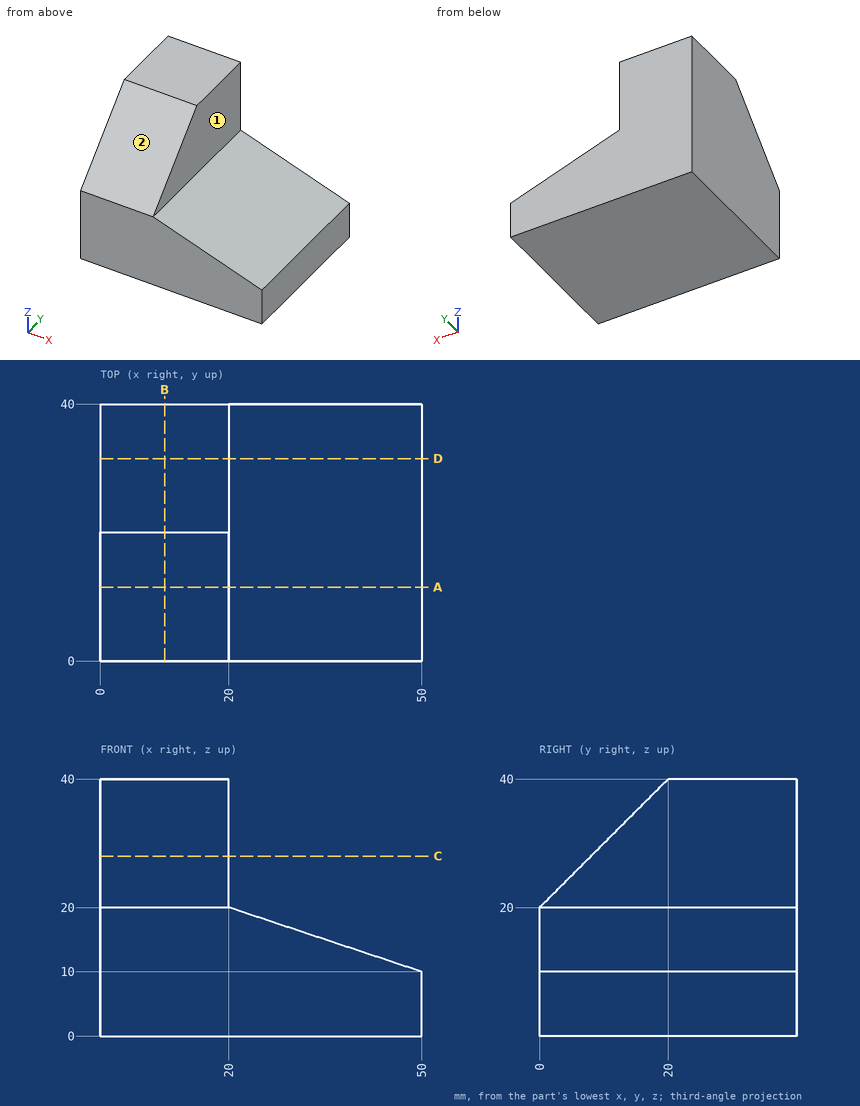
Drawing for the job (mm, zero at the part's lowest x, y, z). A direction names the side the tool comes from. Give positions to 0.01 mm unless a question says otherwise; leave off trailing zeros. Write each loop counter-clockwise with the first axis right and the second up, starting at its lowest first coordinate (ties: lowest second). Pieces come first, ordered by that corner, then holes. Notation, with made-up numbers: (11.25, 40.25) -> (38.25, 40.25) arc R4 cw to (38.25, 46.25) -> close; hole circle Ø1 at (11, 75.25). An arc over 180 degrees is marked (long way). Put each result on its own line as item: value. Start each with the question number.
Item 1: Which spindle directions (+Z, -Z, +X, -X, +Y, -Y) get a long thin tool onto all of the face, cutting with end or side? Do the marked faces 1 and 2. Say none if no direction does.
Item 2: Cut at D-D (y = 31.5). List the corners of the cut face in (x, z), then the cut area to 3 significant figures.
Item 3: Pin check, flat tips, straight feed: pin 1 Ø12 at (x, z) = (11.5, 30.5) entering from -Y; pin 2 Ø5 at (y, z) = (16, 24) entering from +X. Stop position of each tip, or through.
Item 4: Cut at A-A (y = 11.5). List the corners of the cut face in (x, z), then the cut area to 3 significant figures.
Item 5: Wall check: L1, parallel to X at y = 29, z = 23; L2, parallel to Y at x = 9, z = 30; L3, parallel to Y at x = 10, z = 21.5. Give the ranges that are in metal, low to high. Write a range as [from, to].
Item 6: Cut at C-C (z = 28). List the corners of the cut face in (x, y).
Item 7: Cut at B-B (x = 10). List the corners of the cut face in (y, z).
Answer list:
1. face 1: +Z, +X, +Y, -Y
1. face 2: +Z, +X, -X, -Y
2. outline: (0, 0) -> (50, 0) -> (50, 10) -> (20, 20) -> (20, 40) -> (0, 40) -> close
2. area: 1,250 mm2
3. pin 1: stops at y = 4.5
3. pin 2: stops at x = 20
4. outline: (0, 0) -> (50, 0) -> (50, 10) -> (20, 20) -> (20, 31.5) -> (0, 31.5) -> close
4. area: 1,080 mm2
5. L1: x = [0, 20]
5. L2: y = [10, 40]
5. L3: y = [1.5, 40]
6. outline: (0, 8) -> (20, 8) -> (20, 40) -> (0, 40) -> close
7. outline: (0, 0) -> (40, 0) -> (40, 40) -> (20, 40) -> (0, 20) -> close
